from build123d import *

# Parameters (mm, degrees)
SADDLE_DEPTH        = 92.15
SKIRT_CUT_X_DEPTH   = 48.875
SKIRT_CUT_X_2_DEPTH = 48.875
BAIL_LEGS_SKETCH_R  = 12.5
BAIL_LEGS_DEPTH     = 19.975
GRIP_BAR_SKETCH_R   = 12.5
GRIP_BAR_DEPTH      = 51.65
ELBOW_X_SKETCH_R    = 12.5
ELBOW_X_ANGLE       = 90
ELBOW_X_SKETCH_2_R  = 12.5
ELBOW_X_2_ANGLE     = 90
M6_SLOTS_X_DEPTH    = 48.875
M6_SLOTS_X_2_DEPTH  = 48.875
BAIL_BASE_X_R       = 8
BAIL_BASE_X_2_R     = 8
RECESS_CORNERS_R    = 2
LAND_CORNERS_R      = 1
ROOF_CORNERS_R      = 3
ROOF_TOP_EDGE_R     = 2
BED_CHAMFER_SIZE    = 0.6


with BuildPart() as part:
    # saddle sketch → saddle (new, symmetric)
    with BuildSketch(Plane(origin=(0, 0, 0), x_dir=(0, 0, -1), z_dir=(1, 0, 0))):
        Polygon((32.3, 47.875), (-12, 47.875), (-12, -47.875), (32.3, -47.875), (32.3, -43.875), (31.3, -42.875), (0, -42.875), (0, -33.215), (-6, -33.215), (-6, 33.215), (0, 33.215), (0, 42.875), (31.3, 42.875), (32.3, 43.875), align=None)
    extrude(amount=SADDLE_DEPTH, both=True)

    # Sketch2 → skirt cut _x (cut, symmetric)
    with BuildSketch(Plane(origin=(0, 0, 0), x_dir=(1, 0, 0), z_dir=(0, 1, 0))):
        Polygon((46, 33.3), (46, 32.3), (68.907419931, 5), (93.15, 5), (93.15, 33.3), align=None)
    extrude(amount=SKIRT_CUT_X_DEPTH, both=True, mode=Mode.SUBTRACT)

    # Sketch3 → skirt cut -x 2 (cut, symmetric)
    with BuildSketch(Plane(origin=(0, 0, 0), x_dir=(1, 0, 0), z_dir=(0, 1, 0))):
        Polygon((-46, 33.3), (-46, 32.3), (-68.907419931, 5), (-93.15, 5), (-93.15, 33.3), align=None)
    extrude(amount=SKIRT_CUT_X_2_DEPTH, both=True, mode=Mode.SUBTRACT)

    # bail legs sketch → bail legs (add, symmetric)
    with BuildSketch(Plane.XY.offset(30.975)):
        with Locations(Location((69.65, 0, 0), (0, 0, 180))):
            Circle(BAIL_LEGS_SKETCH_R)
        with Locations(Location((-69.65, 0, 0), (0, 0, 180))):
            Circle(BAIL_LEGS_SKETCH_R)
    extrude(amount=BAIL_LEGS_DEPTH, both=True)



with BuildPart() as body_2:
    # grip bar sketch → grip bar (new, symmetric)
    with BuildSketch(Plane(origin=(0, 0, 0), x_dir=(0, 0, -1), z_dir=(1, 0, 0))):
        with Locations((-68.95, 0)):
            Circle(GRIP_BAR_SKETCH_R)
    extrude(amount=GRIP_BAR_DEPTH, both=True)


with BuildPart() as part_1:
    add(part.part)

    add(body_2.part)  # elbow _x merges body 2
    # elbow _x sketch → elbow _x (revolve)
    with BuildSketch(Plane(origin=(51.65, 0, 0), x_dir=(0, 0, -1), z_dir=(1, 0, 0))):
        with Locations(Location((-68.95, 0, 0), (0, 0, 180))):
            Circle(ELBOW_X_SKETCH_R)
    revolve(axis=Axis((51.65, -30, 50.95), (0, 1, 0)), revolution_arc=ELBOW_X_ANGLE)

    # elbow -x sketch 2 → elbow -x 2 (revolve)
    with BuildSketch(Plane(origin=(-51.65, 0, 0), x_dir=(0, 0, -1), z_dir=(1, 0, 0))):
        with Locations(Location((-68.95, 0, 0), (0, 0, 180))):
            Circle(ELBOW_X_SKETCH_2_R)
    revolve(axis=Axis((-51.65, -30, 50.95), (0, -1, 0)), revolution_arc=ELBOW_X_2_ANGLE)

    # Sketch9 → M6 slots _x (cut, symmetric)
    with BuildSketch(Plane(origin=(0, 0, 0), x_dir=(1, 0, 0), z_dir=(0, 1, 0))):
        with BuildLine():
            Line((25.605, 22.3), (25.605, 20.3))
            ThreePointArc((25.605, 20.3), (29.605, 16.3), (33.605, 20.3))
            Line((33.605, 20.3), (33.605, 22.3))
            ThreePointArc((33.605, 22.3), (29.605, 26.3), (25.605, 22.3))
        make_face()
    extrude(amount=M6_SLOTS_X_DEPTH, both=True, mode=Mode.SUBTRACT)

    # Sketch10 → M6 slots -x 2 (cut, symmetric)
    with BuildSketch(Plane(origin=(0, 0, 0), x_dir=(1, 0, 0), z_dir=(0, 1, 0))):
        with BuildLine():
            Line((-33.605, 22.3), (-33.605, 20.3))
            ThreePointArc((-33.605, 20.3), (-29.605, 16.3), (-25.605, 20.3))
            Line((-25.605, 20.3), (-25.605, 22.3))
            ThreePointArc((-25.605, 22.3), (-29.605, 26.3), (-33.605, 22.3))
        make_face()
    extrude(amount=M6_SLOTS_X_2_DEPTH, both=True, mode=Mode.SUBTRACT)

    # bail base _x
    bail_base_x_edges = [part_1.edges().sort_by_distance(p)[0] for p in [
        (82.15, 0, 12),
    ]]
    fillet(bail_base_x_edges, radius=BAIL_BASE_X_R)

    # bail base -x 2
    bail_base_x_2_edges = [part_1.edges().sort_by_distance(p)[0] for p in [
        (-57.15, 0, 12),
    ]]
    fillet(bail_base_x_2_edges, radius=BAIL_BASE_X_2_R)

    # recess corners
    recess_corners_edges = [part_1.edges().sort_by_distance(p)[0] for p in [
        (0, 33.215, 6),
        (0, -33.215, 6),
    ]]
    fillet(recess_corners_edges, radius=RECESS_CORNERS_R)

    # land corners
    land_corners_edges = [part_1.edges().sort_by_distance(p)[0] for p in [
        (0, 42.875, 0),
        (0, -42.875, 0),
    ]]
    fillet(land_corners_edges, radius=LAND_CORNERS_R)

    # roof corners
    roof_corners_edges = [part_1.edges().sort_by_distance(p)[0] for p in [
        (92.15, -47.875, 3.5),
        (-92.15, -47.875, 3.5),
        (92.15, 47.875, 3.5),
        (-92.15, 47.875, 3.5),
    ]]
    fillet(roof_corners_edges, radius=ROOF_CORNERS_R)

    # roof top edge
    roof_top_edge_edges = [part_1.edges().sort_by_distance(p)[0] for p in [
        (0, -47.875, 12),
        (-92.15, 0, 12),
        (92.15, 0, 12),
        (0, 47.875, 12),
        (91.271320344, 46.996320344, 12),
        (91.271320344, -46.996320344, 12),
        (-91.271320344, 46.996320344, 12),
        (-91.271320344, -46.996320344, 12),
    ]]
    fillet(roof_top_edge_edges, radius=ROOF_TOP_EDGE_R - 0.0001)  # a hair under: the kernel refuses the full size

    # bed chamfer
    bed_chamfer_edges = [part_1.edges().sort_by_distance(p)[0] for p in [
        (0, -47.875, -32.3),
        (0, 47.875, -32.3),
    ]]
    chamfer(bed_chamfer_edges, length=BED_CHAMFER_SIZE)


solid = part_1.part
For this review, take the finished solid that the model builds, in its own axes (mm). A direction names the side the tool comes from. Round coordinates to 2 decimals unless told otherwise and drop trailing zeros. Loops run counter-clockwise (first coordinate to the right, second up) from the corner with the lowest first, then second, coordinate; pieces in that order, holes last. Notation, with made-up numbers: (23.25, -18.75) - (62.25, -18.75) arc R28 ccw to (62.25, -0.75) - close; hole circle Ø8 at (88, -11.5). An arc over 180 degrees is marked (long way). Put each result on its own line as item: value. Start each with the question number.
1. Consider section A-A on x = -8.5. State the section outline as (y, z) points (3 decimals), plus the area to 3 significant figures.
2. Mouldability with a two-part tool opening along Y and no side actions: class faces 1 (the flat face through (1, 47.875, -7)), 2 (the flat face through (1, -33.215, 2)), 3 (the cylindrical face through (-29.7, -45.3, -16.3)) as +Y half, -Y half, draft (parallel to the pull), parting line (faces both ways), or undercut.
3. Consider section B-B on z = 22.5. State the section outline as (x, y) points.
4. Insertion check: P1, Ø2.5, axis at x = 77, y = 44, coming from the -Z side; P2, Ø1.6, axis at y = 45, z = -21, coming from the -X side; P3, Ø10, axis at y = -11.5, z = 50, coming from the -X side. Each pin has a flat end and moves straight along its axis. Give the tip position at first contact, or say it passes through.
5. For faces 4 (the flat face through (-80, 45, -5)), 5 (the flat face through (1, 33.215, 2)), 6 (the flat face through (80, -45, -5)), list the 3-axis set-ups (+Z, -Z, +X, -X, +Y, -Y) from which the entire face can be reached by the end or side of a thin tool; tool diameter is ignored.
6. For probe 1 along Y at (x, z) = (31.5, -10.5) (3 decimals); probe 2 along Z at (x, y) = (-44.5, -35.5); probe 3 along Z at (x, y) = (77, 26.5), list the stretches that pass through material, from the lowest coordinate up. Write a range as [from, to].
Result sheet:
1. outline: (-47.875, -31.7) - (-47.275, -32.3) - (-43.875, -32.3) - (-42.875, -31.3) - (-42.875, -1) arc R1 cw to (-41.875, 0) - (-33.215, 0) - (-33.215, 4) arc R2 cw to (-31.215, 6) - (31.215, 6) arc R2 cw to (33.215, 4) - (33.215, 0) - (41.875, 0) arc R1 cw to (42.875, -1) - (42.875, -31.3) - (43.875, -32.3) - (47.275, -32.3) - (47.875, -31.7) - (47.875, 10) arc R2 ccw to (45.875, 12) - (-45.875, 12) arc R2 ccw to (-47.875, 10) - close; circle Ø25 at (0, 68.95)
1. area: 1,560 mm^2
2. face 1: +Y half
2. face 2: undercut
2. face 3: draft
3. outline: circle Ø25 at (-69.65, 0); circle Ø25 at (69.65, 0)
4. P1: z = -5
4. P2: x = -56.15
4. P3: x = -80.33
5. face 4: -Z, -X, +Y, -Y
5. face 5: -Z, +X, -X
5. face 6: -Z, +X, +Y, -Y
6. probe 1: [-47.875, -42.875], [42.875, 47.875]
6. probe 2: [0, 12]
6. probe 3: [6, 12]
